from build123d import *

# Parameters (mm, degrees)
ESQUISSE2_R        = 2.1
BOSS_EXTRU_1_DEPTH = 20.5
ESQUISSE3_W        = 3
ESQUISSE3_H        = 4
BOSS_EXTRU_2_DEPTH = 4.5


with BuildPart() as part:
    # Esquisse1 → Révolution1 (revolve)
    with BuildSketch(Plane.XY, mode=Mode.PRIVATE) as r_volution1_sk:
        with BuildLine():
            Line((0, 33.5), (0, -32.5))
            Line((0, -32.5), (12.1, -32.5))
            Line((12.1, -32.5), (12.1, -1))
            ThreePointArc((12.1, -1), (11.807106781, -0.292893219), (11.1, 0))
            Line((11.1, 0), (13.5, 0))
            Line((13.5, 0), (13.5, 27))
            Line((13.5, 27), (2.1, 27))
            Line((2.1, 27), (2.1, 33.5))
            Line((2.1, 33.5), (0, 33.5))
        make_face()
    revolve(r_volution1_sk.sketch.rotate(Axis((0, 44.171548117, 0), (0, -1, 0)), 90), axis=Axis((0, 44.171548117, 0), (0, -1, 0)))

    # Esquisse2 → Boss.-Extru.1 (add)
    with BuildSketch(Plane.XY):
        with Locations(Location((0, 5.8, 0), (0, 0, 90))):
            Circle(ESQUISSE2_R)
    extrude(amount=BOSS_EXTRU_1_DEPTH)

    # Esquisse3 → Boss.-Extru.2 (add)
    with BuildSketch(Plane.XZ.offset(32.5)):
        with Locations((-9, 0)):
            Rectangle(ESQUISSE3_W, ESQUISSE3_H)
        with Locations((9, 0)):
            Rectangle(ESQUISSE3_W, ESQUISSE3_H)
    extrude(amount=BOSS_EXTRU_2_DEPTH)


solid = part.part
Build history of the part. All positions in model axes, mm. A direction names the side the tool comes from. Round coordinates to 2 decimals unless told otherwise and drop trailing zeros. Order: outer loops, then holes, each group sorted by start corner. A loop starts at its lowest first (then second) coordinate and runs counter-clockwise, first axis right, second up. Notation, with made-up numbers: M 2,37 L 50,37 A27 cw 50,72 Z; hole C -24,23 d6. An arc over 180 degrees is marked long. Use CSV: the item, a comma, the result in double quotes. Start each with the question number.
(1) Cut at C-C on y = 5.8. List the corners of the cut face in (x, z), then the cut area to 3 significant figures.
(2) Tool access for faces 1 (the face through (-3.635, -16.53, 11.541)), 2 (the face through (-10.5, -35, 0)), 3 (the face through (10.5, -35, 0)), 4 (the face through (-7.5, -35, 0)), 5 (the face through (-9, -35, 2)): list every direction of +Z, -Z, +X, -X, +Y, -Y with a clear straight run to the whole face (end or side of a thin tool).
(3) Flat gauge pins, fed straight in: P1, Ø2.5, axis at x = 8.5, y = -34, coming from the -Z side; P2, Ø10, axis at x = 6.5, z = -10, coming from the -Y side; P3, Ø1.2, axis at y = -35.5, z = -0.5, coming from the -X side. Where does each tip first touch, or does it go through?
(4) Drill centre lines: probe 1 along Y at (x, z) = (2, 0); probe 2 along Y at (x, z) = (6, 6); probe 3 along Z at (x, y) = (6, -9). Where is each one in solid material? Low to high.
(5) Cut at A-A on x = 0. List the corners of the cut face in (y, z), then the cut area to 3 significant figures.
(6) Cut at B-B on z = 0. List the corners of the cut face in (x, y).
(7) Cut at D-D on y = -29. List the corners of the cut face in (x, z).
Findings:
1,outline,"M -2.1,13.34 A13.5 ccw long 2.1,13.34 L 2.1,20.5 L -2.1,20.5 Z"
1,area,"602 mm^2"
2,face 1,"-Y"
2,face 2,"+Z, -Z, -X, -Y"
2,face 3,"+Z, -Z, +X, -Y"
2,face 4,"+Z, -Z, -Y"
2,face 5,"+Z, +X, -X, -Y"
3,P1,"stops at z = -2"
3,P2,"stops at y = -32.5"
3,P3,"stops at x = -10.5"
4,probe 1,"y = -32.5 to 33.5"
4,probe 2,"y = -32.5 to 27"
4,probe 3,"z = -10.51 to 10.51"
5,outline,"M -32.5,-12.1 L -1,-12.1 A1 ccw 0,-11.1 L 0,-13.5 L 27,-13.5 L 27,-2.1 L 33.5,-2.1 L 33.5,2.1 L 27,2.1 L 27,13.5 L 7.9,13.5 L 7.9,20.5 L 3.7,20.5 L 3.7,13.5 L 0,13.5 L 0,11.1 A1 ccw -1,12.1 L -32.5,12.1 Z"
5,area,"1,570 mm^2"
6,outline,"M -13.5,0 L -11.1,0 A1 ccw -12.1,-1 L -12.1,-32.5 L -10.5,-32.5 L -10.5,-37 L -7.5,-37 L -7.5,-32.5 L 7.5,-32.5 L 7.5,-37 L 10.5,-37 L 10.5,-32.5 L 12.1,-32.5 L 12.1,-1 A1 ccw 11.1,0 L 13.5,0 L 13.5,27 L 2.1,27 L 2.1,33.5 L -2.1,33.5 L -2.1,27 L -13.5,27 Z"
7,outline,"C 0,0 d24.2"
